```python
from build123d import *

# Parameters (mm, degrees)
F0_R     = 6
F1_DEPTH = 24
F0_R_2   = 9.9999997765
F2_DEPTH = 2
F3_R     = 4
F4_DEPTH = 22


with BuildPart() as f1:
    # F0 (on Front) → F1 (new body)
    with BuildSketch(Plane.XZ):
        Circle(F0_R)
    extrude(amount=F1_DEPTH)

    # F0 (on Front) → F2 (join)
    with BuildSketch(Plane.XZ):
        Circle(F0_R_2)
        Circle(F0_R, mode=Mode.SUBTRACT)
    extrude(amount=F2_DEPTH)

    # F3
    f3_edges = [f1.edges().sort_by_distance(p)[0] for p in [
        (-6, -24, 0),
    ]]
    fillet(f3_edges, radius=F3_R)

    # F4 (cut): a face of the model
    f4_faces = [f1.faces().sort_by_distance(p)[0] for p in [
        (0, -24, 0),
    ]]
    extrude(f4_faces, amount=-F4_DEPTH, mode=Mode.SUBTRACT)


solid = f1.part
```
Design review of the part built by this model. Coordinates are the model's own, in mm. Coordinates: 2 decimals unless noted, no trailing zeros. Loops run counter-clockwise (first coordinate to the right, second up) from the corner with the lowest first, then second, coordinate; pieces in that order, holes last. Notation, with made-up numbers: (8.5, 6.25) - (43.5, 6.25) arc R16 cw to (43.5, 10.25) - close; hole circle Ø9 at (44.5, 53.25). An arc over 180 degrees is marked (long way). Use CSV: the item, a comma, the result in double quotes. Start each with the question number.
1) Consider section B-B on z = 7.5. Write out the cut boundary in (x, y), then the cut area to 3 significant figures.
2) Wall thickness on L1, parallel to Z at x = 0, y = -7.75; L2, parallel to Y at x = -1, z = -0.5; L3, parallel to Z at x = 1.75, y = -2.5: over which ranges is each line inside the solid? List them lowest first. Write a range as from..to.
3) For pin 1 Ø1.5 at (y, z) = (-16.5, -1) entering from +X; pin 2 Ø8 at (y, z) = (-7, -7.5) entering from +X; pin 3 Ø10 at (x, z) = (-7.5, -1.5) entering from -Y, all flat-tipped, find the tip position at first contact; note any pin that passes through.
4) The part is to be moulded in two halves that separate along Z. For faces 1 (the flat face through (0, -2, 0)), 2 (the flat face through (0, 0, 0)), 3 (the cylindrical face through (-2.17, -0.99, -9.76)), say which applies: +Z half, -Z half, draft (parallel to the pull), parting line (faces both ways), or undercut.
5) Consider section A-A on y = -8.75. Write out the cut boundary in (x, z).
Geometry says:
1,outline,"(-6.61, -2) - (6.61, -2) - (6.61, 0) - (-6.61, 0) - close"
1,area,"26.5 mm^2"
2,L1,"-6..-2, 2..6"
2,L2,"-2..0"
2,L3,"-5.74..-0.97, 0.97..5.74"
3,pin 1,"x = 5.99"
3,pin 2,"x = 4.87"
3,pin 3,"y = -23.95"
4,face 1,"undercut"
4,face 2,"draft"
4,face 3,"parting line"
5,outline,"circle Ø12 at (0, 0); hole circle Ø4 at (0, 0)"
